from build123d import *

# Parameters (mm, degrees)
ESBO_O1_R                            = 2.5
ESBO_O1_R_2                          = 1.5
RESSALTO_EXTRUS_O3_DEPTH             = 1.5
ESBO_O2_R                            = 5.125
RESSALTO_EXTRUS_O4_DEPTH             = 5
RESSALTO_EXTRUS_O4_DIRECTION_2_REACH = 64.207
ESBO_O3_R                            = 4.125
CORTE_EXTRUS_O1_DEPTH                = 10
FILETE1_R                            = 5


with BuildPart() as part:
    # Esboço1 → Ressalto-extrusão3 (new, symmetric)
    with BuildSketch(Plane.XY):
        with BuildLine():
            Line((3, -3), (12.5, -3))
            ThreePointArc((12.5, -3), (15.5, 0), (12.5, 3))
            Line((12.5, 3), (3, 3))
            Line((3, 3), (3, 12.5))
            ThreePointArc((3, 12.5), (0, 15.5), (-3, 12.5))
            Line((-3, 12.5), (-3, 3))
            Line((-3, 3), (-57.17, 3))
            ThreePointArc((-57.17, 3), (-60.17, 0), (-57.17, -3))
            Line((-57.17, -3), (-3, -3))
            Line((-3, -3), (-3, -12.5))
            ThreePointArc((-3, -12.5), (0, -15.5), (3, -12.5))
            Line((3, -12.5), (3, -3))
        make_face()
        Circle(ESBO_O1_R, mode=Mode.SUBTRACT)
        with Locations((-12.5, 0)):
            Circle(ESBO_O1_R_2, mode=Mode.SUBTRACT)
        with Locations((0, 12.5)):
            Circle(ESBO_O1_R_2, mode=Mode.SUBTRACT)
        with Locations((12.5, 0)):
            Circle(ESBO_O1_R_2, mode=Mode.SUBTRACT)
        with Locations((0, -12.5)):
            Circle(ESBO_O1_R_2, mode=Mode.SUBTRACT)
    extrude(amount=RESSALTO_EXTRUS_O3_DEPTH, both=True)

    # Esboço2 → Ressalto-extrusão4 (add)
    with BuildSketch(Plane.XY.offset(1.5)):
        with Locations((-57.17, 0)):
            Circle(ESBO_O2_R)
    extrude(amount=RESSALTO_EXTRUS_O4_DEPTH)

    # Ressalto-extrusão4 direction 2: up to this face of the body (flat: up to its plane)
    ressalto_extrus_o4_direction_2_end = Plane(part.part.faces().sort_by_distance((-18.436716942, 0, -1.5))[0])
    # Esboço2 → Ressalto-extrusão4 direction 2 (add, up to the picked face)
    with BuildSketch(Plane.XY.offset(1.5), mode=Mode.PRIVATE) as ressalto_extrus_o4_direction_2_sk1:
        with Locations((-57.17, 0)):
            Circle(ESBO_O2_R)
    ressalto_extrus_o4_direction_2_tool1 = split(extrude(ressalto_extrus_o4_direction_2_sk1.sketch, amount=-RESSALTO_EXTRUS_O4_DIRECTION_2_REACH, mode=Mode.PRIVATE), bisect_by=ressalto_extrus_o4_direction_2_end, keep=Keep.BOTH, mode=Mode.PRIVATE)
    add(ressalto_extrus_o4_direction_2_tool1.solids().sort_by(Axis((-57.17, 0, 1.5), (0, 0, -1)))[0])

    # Esboço3 → Corte-extrusão1 (cut)
    with BuildSketch(Plane.XY.offset(6.5)):
        with Locations((-57.17, 0)):
            Circle(ESBO_O3_R)
    extrude(amount=-CORTE_EXTRUS_O1_DEPTH, mode=Mode.SUBTRACT)

    # Filete1
    filete1_edges = [part.edges().sort_by_distance(p)[0] for p in [
        (3, -3, 0),
        (-3, -3, 0),
        (-3, 3, 0),
        (3, 3, 0),
        (-53.014807465, -3, 0),
        (-53.014807465, 3, 0),
    ]]
    fillet(filete1_edges, radius=FILETE1_R)


solid = part.part
Design review of the part built by this model. Coordinates are the model's own, in mm. A direction names the side the tool comes from. Coordinates: 2 decimals unless noted, no trailing zeros. Loops run counter-clockwise (first coordinate to the right, second up) from the corner with the lowest first, then second, coordinate; pieces in that order, holes last. Notation, with made-up numbers: (5.25, 15) -> (34.25, 15) arc R24 ccw to (34.25, 34) -> close; hole circle Ø7 at (-14, -20.5). An arc over 180 degrees is marked (long way). Use a Markdown table: item, result. Add a question column.
Item 1: Wall thickness on L1, parallel to Y at x = 0, z = 0.2; L2, parallel to X at y = 9.5, z = -1; L3, parallel to Y at x = -12.5, z = 0.7: over which ranges is each line inside the solid? List them lowest first. Write a range as from..to.
Item 2: We need section A-A, the plane y = 0. Write out the cut boundary in (x, z) (3 decimals).
Item 3: Clearance check with flat-ended pins moving along their axes: P1, Ø2.5, axis at x = 0, y = -12.5, coming from the -Z side; P2, Ø1.5, axis at y = -10, z = 0.5, coming from the -X side; P3, Ø1.5, axis at y = -2.5, z = 2.5, coming from the +X side; P4, Ø5, axis at x = -12.5, y = 0, coming from the -Z side. State where each tip first meets the part, or that it passes through.
Item 4: Machinability: for faces 5 (the flat face through (-3, -10, 0)), 6 (the flat face through (10, 3, 0)), 7 (the cylindrical face through (-52.61, -3.28, 0.02)), 8 (the flat face through (-29, 3, 0)), which of the approach directions +Z, -Z, +X, -X, +Y, -Y give a long, thin tool a straight path to every point of the face, cutting with its end or side? Answer none if there is none.
Item 5: We need section B-B, the plane x = -57.17. Write out the cut boundary in (y, z) (3 decimals).
Item 6: The part is to be moulded in two halves that separate along Y. For faces 1 (the cylindrical face through (-0.1, -15.5, 0)), 2 (the cylindrical face through (15.5, -0.1, 0)), 3 (the cylindrical face through (-14, 0, 0)), 4 (the flat face through (3, -10, 0)), say which applies: +Y half, -Y half, draft (parallel to the pull), parting line (faces both ways), or undercut.
Item 7: We need section D-D, the plane x = -47. Write out the cut boundary in (y, z), and give its area (3 significant figures).
Item 8: We need section C-C, the plane z = 3.5. Write out the cut boundary in (x, y) (3 decimals), and give its area (3 significant figures).
Numbers:
| question | item | result |
|---|---|---|
| 1 | L1 | y = -15.5..-14, -11..-2.5, 2.5..11, 14..15.5 |
| 1 | L2 | x = -3..3 |
| 1 | L3 | y = -3..-1.5, 1.5..3 |
| 2 | outline | (-62.295, -1.5) -> (-61.295, -1.5) -> (-61.295, 6.5) -> (-62.295, 6.5) -> close; (-53.045, -1.5) -> (-14, -1.5) -> (-14, 1.5) -> (-52.045, 1.5) -> (-52.045, 6.5) -> (-53.045, 6.5) -> close; (-11, -1.5) -> (-2.5, -1.5) -> (-2.5, 1.5) -> (-11, 1.5) -> close; (2.5, -1.5) -> (11, -1.5) -> (11, 1.5) -> (2.5, 1.5) -> close; (14, -1.5) -> (15.5, -1.5) -> (15.5, 1.5) -> (14, 1.5) -> close |
| 3 | P1 | passes through |
| 3 | P2 | stops at x = -3 |
| 3 | P3 | stops at x = -52.35 |
| 3 | P4 | stops at z = -1.5 |
| 4 | face 5 | +Z, -Z, -X, -Y |
| 4 | face 6 | +Z, -Z, +X, +Y |
| 4 | face 7 | +Z, -Z, -Y |
| 4 | face 8 | +Z, -Z, +Y |
| 5 | outline | (-5.125, -1.5) -> (-4.125, -1.5) -> (-4.125, 6.5) -> (-5.125, 6.5) -> close; (4.125, -1.5) -> (5.125, -1.5) -> (5.125, 6.5) -> (4.125, 6.5) -> close |
| 6 | face 1 | -Y half |
| 6 | face 2 | parting line |
| 6 | face 3 | undercut |
| 6 | face 4 | draft |
| 7 | outline | (-3, -1.5) -> (3, -1.5) -> (3, 1.5) -> (-3, 1.5) -> close |
| 7 | area | 18.0 mm^2 |
| 8 | outline | circle Ø10.25 at (-57.17, 0); hole circle Ø8.25 at (-57.17, 0) |
| 8 | area | 29.1 mm^2 |
